from build123d import *

# Parameters (mm, degrees)
PAD_DEPTH       = 2.25
POCKET_DEPTH    = 5
PAD009_DEPTH    = 2
FILLET003_R     = 0.5
CHAMFER001_SIZE = 3
FILLET004_R     = 1
FILLET008_R     = 0.5
FILLET009_R     = 3


with BuildPart() as part:
    # Sketch → Pad (new body)
    with BuildSketch(Plane.XY):
        Polygon((-0.972695, 0), (3.027305, 0), (3.027305, 4), (35.027305, 4), (35.027305, 0), (39.027305, 0), (39.027305, 15), (-0.972695, 15), align=None)
    extrude(amount=PAD_DEPTH)

    # Sketch002 → Pocket (cut)
    with BuildSketch(Plane.XY.offset(2.25)):
        with BuildLine():
            ThreePointArc((2.744542, 13), (1.027305, 11.282763), (2.744542, 9.565525))
            Line((2.744542, 9.565525), (35.310067, 9.565525))
            ThreePointArc((35.310067, 9.565525), (37.027305, 11.282763), (35.310067, 13))
            Line((2.744542, 13), (35.310067, 13))
        make_face()
    extrude(amount=-POCKET_DEPTH, mode=Mode.SUBTRACT)

    # Sketch012 (on Face5 of Pocket) → Pad009 (join)
    with BuildSketch(Plane.XY.offset(2.25)):
        Polygon((-0.972695, 0), (3.027305, 0), (3.027305, 4), (35.027305, 4), (35.027305, 0), (39.027305, 0), (39.027305, 6.433802), (-0.972695, 6.433802), align=None)
    extrude(amount=PAD009_DEPTH)

    # Fillet003
    fillet003_edges = [part.edges().sort_by_distance(p)[0] for p in [
        (3.027305, 0, 1.125),
        (3.027305, 0, 3.25),
        (35.027305, 0, 1.125),
        (35.027305, 0, 3.25),
    ]]
    fillet(fillet003_edges, radius=FILLET003_R)

    # Chamfer001
    chamfer001_edges = [part.edges().sort_by_distance(p)[0] for p in [
        (-0.972695, 0, 1.125),
        (-0.972695, 0, 3.25),
        (39.027305, 0, 1.125),
        (39.027305, 0, 3.25),
    ]]
    chamfer(chamfer001_edges, length=CHAMFER001_SIZE)

    # Fillet004
    fillet004_edges = [part.edges().sort_by_distance(p)[0] for p in [
        (39.027305, 3, 3.25),
        (39.027305, 3, 1.125),
        (-0.972695, 3, 3.25),
        (-0.972695, 3, 1.125),
    ]]
    fillet(fillet004_edges, radius=FILLET004_R)

    # Fillet008
    fillet008_edges = [part.edges().sort_by_distance(p)[0] for p in [
        (0.673752, 1.353553, 4.25),
        (2.277305, 0, 4.25),
        (2.880858, 0.146447, 4.25),
        (3.027305, 2.25, 4.25),
        (-0.896575, 3.03153, 4.25),
        (-0.972695, 4.924008, 4.25),
        (35.027305, 2.25, 4.25),
        (35.173752, 0.146447, 4.25),
        (35.777305, 0, 4.25),
        (37.380858, 1.353553, 4.25),
        (38.951184, 3.03153, 4.25),
        (39.027305, 4.924008, 4.25),
    ]]
    fillet(fillet008_edges, radius=FILLET008_R)

    # Fillet009
    fillet009_edges = [part.edges().sort_by_distance(p)[0] for p in [
        (-0.972695, 15, 1.125),
        (39.027305, 15, 1.125),
    ]]
    fillet(fillet009_edges, radius=FILLET009_R)


with BuildPart() as part_1:
    # Body placement: moved
    add(part.part.moved(Location((30, -12.6, 3))))


solid = part_1.part
Build history of the part. All positions in model axes, mm. A direction names the side the tool comes from. Round coordinates to 2 decimals unless told otherwise and drop trailing zeros. Write each loop counter-clockwise with the first axis right and the second up, starting at its lowest first coordinate (ties: lowest second). Pieces come first, ordered by that corner, then holes. Notation, with made-up numbers: (64.25, 79.5) -> (95.25, 79.5) arc R32 ccw to (95.25, 111.5) -> close; hole circle Ø1 at (43, -8.75). An arc over 180 degrees is marked (long way). Write item = value, one per line.
(1) Tool access for faces 1 (the face through (49, -8.6, 5)), 2 (the face through (69.027, -6, 4)), 3 (the face through (30.655, -11.227, 4.901)), 4 (the face through (49, -4, 5.25)), 5 (the face through (49, -3.034, 4)): list every direction of +Z, -Z, +X, -X, +Y, -Y with a clear straight run to the whole face (end or side of a thin tool).
Answer:
face_1 = +Z, -Z, -Y
face_2 = +Z, -Z, +X, +Y, -Y
face_3 = +Z, -Z, -X, -Y
face_4 = +Z, +X, -X, +Y
face_5 = +Z, -Z
(2) Band-saw the part on A-A (z = 3.7). Give the cut face in (x, y).
Answer:
outline = (29.03, -9.19) arc R1 ccw to (29.32, -9.89) -> (32.03, -12.6) -> (32.53, -12.6) arc R0.5 ccw to (33.03, -12.1) -> (33.03, -8.6) -> (65.03, -8.6) -> (65.03, -12.1) arc R0.5 ccw to (65.53, -12.6) -> (66.03, -12.6) -> (68.73, -9.89) arc R1 ccw to (69.03, -9.19) -> (69.03, -0.6) arc R3 ccw to (66.03, 2.4) -> (32.03, 2.4) arc R3 ccw to (29.03, -0.6) -> close; hole (32.74, -3.03) -> (65.31, -3.03) arc R1.72 ccw to (65.31, 0.4) -> (32.74, 0.4) arc R1.72 ccw to start
(3) Flat gauge pins, fed straight in: pin 1 (1.5 mm diameter, centred on x = 41.5, z = 6, fed in from -Y); pin 2 (1.5 mm diameter, centred on y = -9.5, z = 6, fed in from +X); pin 3 (2 mm diameter, centred on x = 39, y = -4, fed in from +Z); pin 4 (1 mm diameter, centred on y = -11, z = 5.5, fed in from -X). Where does each tip first touch, or does it go through?
Answer:
pin_1 = -8.6
pin_2 = 69.03
pin_3 = 5.25
pin_4 = 29.93
(4) Probe L1, parallel to X at y = -8.75, z = 4.25; L2, parallel to Y at x = 55.5, z = 5.2; L3, parallel to Y at x = 60, z = 5.75. List the from-to ranges inside material, lowest first.
Answer:
L1 = 29.03 to 33.03, 65.03 to 69.03
L2 = -8.6 to -3.03, 0.4 to 2.4
L3 = -8.6 to -6.17
(5) Band-saw the part on D-D (z = 6.35). Give the cut face in (x, y), then the cut area to 3 significant figures.
Answer:
outline = (29.03, -9.19) arc R1 ccw to (29.32, -9.89) -> (32.03, -12.6) -> (32.53, -12.6) arc R0.5 ccw to (33.03, -12.1) -> (33.03, -8.6) -> (65.03, -8.6) -> (65.03, -12.1) arc R0.5 ccw to (65.53, -12.6) -> (66.03, -12.6) -> (68.73, -9.89) arc R1 ccw to (69.03, -9.19) -> (69.03, -6.17) -> (29.03, -6.17) -> close
area = 120 mm2
(6) Two-plate mould, pull along X, no slides. Class faces 6 (the face through (49, -8, 7.25)), 7 (the face through (29.027, -6, 4)), 8 (the face through (67.027, -1.355, 4.141)), 9 (the face through (67.36, -11.27, 4.85)): pulls with the +X half, pulls with the -X half, needs draft (parallel to the pull), parting line crosses it, or undercut.
Answer:
face_6 = needs draft
face_7 = pulls with the -X half
face_8 = undercut
face_9 = pulls with the +X half
(7) Band-saw the part on B-B (x = 38). Give the cut face in (y, z), then the cut area to 3 significant figures.
Answer:
outline = (-8.6, 3) -> (-3.03, 3) -> (-3.03, 5.25) -> (-6.17, 5.25) -> (-6.17, 7.25) -> (-8.6, 7.25) -> close; (0.4, 3) -> (2.4, 3) -> (2.4, 5.25) -> (0.4, 5.25) -> close
area = 21.9 mm2
(8) Band-saw the part on C-C (y = 0). Give the cut face in (x, z).
Answer:
outline = (29.09, 3) -> (31.64, 3) -> (31.64, 5.25) -> (29.09, 5.25) -> close; (66.41, 3) -> (68.97, 3) -> (68.97, 5.25) -> (66.41, 5.25) -> close
